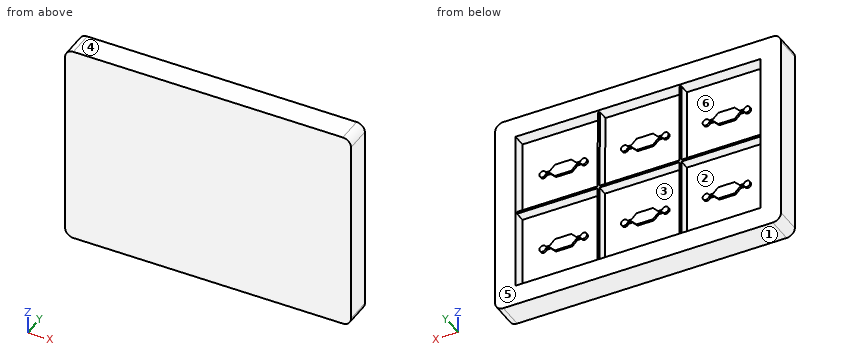
```python
from build123d import *

# Parameters (mm, degrees)
SKETCH1_W            = 70
SKETCH1_H            = 50
BOSS_EXTRUDE1_DEPTH  = 6.35
SKETCH2_W            = 60
SKETCH2_H            = 40
CUT_EXTRUDE1_DEPTH   = 3.175
DIVIDERS_DEPTH       = 2.5
BOSS_EXTRUDE3_DEPTH  = 0.5
LPATTERN1_COUNT      = 3
LPATTERN1_PITCH      = 20
LPATTERN1_COUNT_DIR2 = 2
LPATTERN1_PITCH_DIR2 = 20
FILLET1_R            = 2


with BuildPart() as part:
    # Sketch1 → Boss-Extrude1 (new body)
    with BuildSketch(Plane(origin=(0, 0, 0), x_dir=(1, 0, 0), z_dir=(0, 1, 0))):
        Rectangle(SKETCH1_W, SKETCH1_H)
    extrude(amount=BOSS_EXTRUDE1_DEPTH)

    # Sketch2 → Cut-Extrude1 (cut)
    with BuildSketch(Plane(origin=(0, 6.35, 0), x_dir=(1, 0, 0), z_dir=(0, 1, 0))):
        Rectangle(SKETCH2_W, SKETCH2_H)
    extrude(amount=-CUT_EXTRUDE1_DEPTH, mode=Mode.SUBTRACT)

    # Sketch10 → Dividers (add)
    with BuildSketch(Plane(origin=(0, 3.175, 0), x_dir=(1, 0, 0), z_dir=(0, 1, 0))):
        Polygon((-10.25, -0.25), (-10.25, -20), (-9.75, -20), (-9.75, -0.25), (9.818560524, -0.25), (9.681439476, -20), (10.181439476, -20), (10.318560524, -0.25), (30, -0.25), (30, 0.25), (10.318560524, 0.25), (10.318560524, 20), (9.818560524, 20), (9.818560524, 0.25), (-9.75, 0.25), (-9.75, 20), (-10.25, 20), (-10.25, 0.25), (-30, 0.25), (-30, -0.25), align=None)
    extrude(amount=DIVIDERS_DEPTH)

    # Sketch11 → Boss-Extrude3 (add)
    with BuildSketch(Plane(origin=(0, 3.175, 0), x_dir=(1, 0, 0), z_dir=(0, 1, 0))):
        with BuildLine():
            Line((-24.464905709, 9.875), (-24.464905709, 10.375))
            ThreePointArc((-24.464905709, 10.375), (-26.024839917, 10.125), (-24.464905709, 9.875))
        make_face()
        Polygon((-24.464905709, 9.875), (-24.464905709, 10.375), (-23.464905709, 10.375), (-22.208630276, 11.631275433), (-18.208630276, 11.631275433), (-16.952354844, 10.375), (-15.952354844, 10.375), (-15.952354844, 9.875), (-16.952354844, 9.875), (-18.208630276, 8.618724567), (-22.208630276, 8.618724567), (-23.464905709, 9.875), align=None)
        with BuildLine():
            Line((-15.952354844, 10.375), (-15.952354844, 9.875))
            ThreePointArc((-15.952354844, 9.875), (-14.392420636, 10.125), (-15.952354844, 10.375))
        make_face()
    boss_extrude3 = extrude(amount=BOSS_EXTRUDE3_DEPTH)

    # LPattern1: Boss-Extrude3 3 × 2
    with Locations(*[(i * LPATTERN1_PITCH, 0, j * LPATTERN1_PITCH_DIR2) for i in range(LPATTERN1_COUNT) for j in range(LPATTERN1_COUNT_DIR2) if (i, j) != (0, 0)]):
        add(boss_extrude3)

    # Fillet1
    fillet1_edges = [part.edges().sort_by_distance(p)[0] for p in [
        (35, 3.175, 25),
        (-35, 3.175, 25),
        (-35, 3.175, -25),
        (35, 3.175, -25),
    ]]
    fillet(fillet1_edges, radius=FILLET1_R)


solid = part.part
```
Design review of the part built by this model. Coordinates are the model's own, in mm. Face numbers are marked on the shaded views. A direction names the side the tool comes from. Coordinates: 2 decimals unless noted, no trailing zeros. Write each loop counter-clockwise with the first axis right and the second up, starting at its lowest first coordinate (ties: lowest second). Pieces come first, ordered by that corner, then holes.
1) Add section A-A (y = 4.75). State how many separate pieces and enclosed holes the cut face has, plus the area to 3 significant figures.
2) Mouldability with a two-part tool opening along Z and no side actions: class the marked faces 3, 4, 5 and 6 as +Z half, -Z half, draft (parallel to the pull), parting line (faces both ways), or undercut.
3) Add section B-B (x = -19.5). Write out the cut boundary in (y, z) (3 decimals), plus the area to 3 significant figures.
4) Add section C-C (z = 18.5). Write out the cut boundary in (x, y) (3 decimals), plus the area to 4 significant figures.
5) Machinability: for the marked faces 1 and 2, which of the approach directions +Z, -Z, +X, -X, +Y, -Y give a long, thin tool a straight path to every point of the face, cutting with its end or side? Answer none if there is none.
6) Add section D-D (x = -7.5). Write out the cut boundary in (y, z) (3 decimals).
7) To check wall thickness, follow L1, parallel to Z at x = 16, y = 3.75; L2, parallel to X at y = 4, z = -8; L3, parallel to X at y = 4, z = 19. State the ranges of each line that lie inside material, in increasing order.
8) Insertion check: pin 1 (8 mm diameter, centred on x = -24.5, z = 2.5, fed in from +Y) (3 decimals); pin 2 (3.5 mm diameter, centred on x = 20.5, z = -11, fed in from +Y) (3 decimals). Each pin has a flat end and moves straight along its axis. Give the tip position at first contact, or say it passes through.
Check result:
1. separate pieces: 1
1. enclosed holes: 6
1. area: 1,170 mm2
2. face 3: undercut
2. face 4: +Z half
2. face 5: draft
2. face 6: undercut
3. outline: (0, -25) - (6.35, -25) - (6.35, -20) - (3.175, -20) - (3.175, -11.631) - (3.675, -11.631) - (3.675, -8.619) - (3.175, -8.619) - (3.175, -0.25) - (5.675, -0.25) - (5.675, 0.25) - (3.175, 0.25) - (3.175, 8.369) - (3.675, 8.369) - (3.675, 11.381) - (3.175, 11.381) - (3.175, 20) - (6.35, 20) - (6.35, 25) - (0, 25) - close
3. area: 195 mm2
4. outline: (-35, 0) - (35, 0) - (35, 6.35) - (30, 6.35) - (30, 3.175) - (10.192, 3.175) - (10.192, 5.675) - (9.692, 5.675) - (9.692, 3.175) - (-9.75, 3.175) - (-9.75, 5.675) - (-10.25, 5.675) - (-10.25, 3.175) - (-30, 3.175) - (-30, 6.35) - (-35, 6.35) - close
4. area: 256.5 mm2
5. face 1: -Z, +X, -X, +Y, -Y
5. face 2: +Y
6. outline: (0, -25) - (6.35, -25) - (6.35, -20) - (3.175, -20) - (3.175, -0.25) - (5.675, -0.25) - (5.675, 0.25) - (3.175, 0.25) - (3.175, 20) - (6.35, 20) - (6.35, 25) - (0, 25) - close
7. L1: z = -25 to -20, -0.25 to 0.25, 20 to 25
7. L2: x = -35 to -30, -10.25 to -9.75, 9.82 to 10.32, 30 to 35
7. L3: x = -35 to -30, -10.25 to -9.75, 9.69 to 10.19, 30 to 35
8. pin 1: stops at y = 5.675
8. pin 2: stops at y = 3.675
